from build123d import *


with BuildPart() as part:
    # 草图1 → 旋转1 (revolve)
    with BuildSketch(Plane.XY):
        with BuildLine():
            Line((0, 0), (0, 2.7))
            ThreePointArc((0, 2.7), (0.087867966, 2.912132034), (0.3, 3))
            Line((0.3, 3), (1.1, 3))
            Line((1.1, 3), (1.1, 1.5))
            Line((1.1, 1.5), (12.1, 1.5))
            Line((12.1, 1.5), (12.1, 3))
            Line((12.1, 3), (12.9, 3))
            ThreePointArc((12.9, 3), (13.112132034, 2.912132034), (13.2, 2.7))
            Line((13.2, 2.7), (13.2, 0))
            Line((13.2, 0), (0, 0))
        make_face()
    revolve(axis=Axis((13.2, 0, 0), (-1, 0, 0)))


solid = part.part
Geometry: final body of the model. Coordinates: model frame, mm. A direction names the side the tool comes from. Coordinates: 2 decimals unless noted, no trailing zeros. Order: outer loops, then holes, each group sorted by start corner. A loop starts at its lowest first (then second) coordinate and runs counter-clockwise, first axis right, second up.
(1) Section query A-A (z = 0). Return the cut outline in (x, y).
(2) Draft query along X for faces 3 (the face through (12.5, -3, -0.1)), 4 (the face through (0, 0, 0)), 5 (the face through (6.68, -1.5, -0.07)), 6 (the face through (13.2, 0, 0)). Return one class per face: pulls with the +X half, pulls with the -X half, needs draft (parallel to the pull), parting line crosses it, or undercut.
(3) Material intervals for probe 1 along X at (y, z) = (0, 2.25); probe 2 along Z at (x, y) = (9, -0.75); probe 3 along Y at (x, z) = (10.25, -0.5), sorted ascending.
(4) Section query C-C (x = 10.25). Return the cut outline in (y, z), plus the area to 3 significant figures.
(5) Access query for faces 1 (the face through (12.1, -1.3, 1.3)), 2 (the face through (0.7, -3, -0.1)). Directions: +Z, -Z, +X, -X, +Y, -Y. A direction counts if a zero-diameter tool reaches every point of the face in a straight line with its end or side. Return the directions, or none.
(6) First-contact query: pin 1 (3 mm diameter, centred on x = 10.5, z = -2.5, fed in from +Y). Flat tip, straight axial feed; report the tip coordinate or a pass-through.
Solution:
1. outline: (0, -2.7) arc R0.3 ccw to (0.3, -3) - (1.1, -3) - (1.1, -1.5) - (12.1, -1.5) - (12.1, -3) - (12.9, -3) arc R0.3 ccw to (13.2, -2.7) - (13.2, 2.7) arc R0.3 ccw to (12.9, 3) - (12.1, 3) - (12.1, 1.5) - (1.1, 1.5) - (1.1, 3) - (0.3, 3) arc R0.3 ccw to (0, 2.7) - close
2. face 3: needs draft
2. face 4: pulls with the -X half
2. face 5: undercut
2. face 6: pulls with the +X half
3. probe 1: x = 0 to 1.1, 12.1 to 13.2
3. probe 2: z = -1.3 to 1.3
3. probe 3: y = -1.41 to 1.41
4. outline: circle Ø3 at (0, 0)
4. area: 7.07 mm2
5. face 1: none
5. face 2: +X, -X
6. pin 1: stops at y = 1.12
